Drawing for the job (mm, zero at the part's lowest x, y, z). A direction names the side the tool comes from. Give positions to 0.01 mm unless a question says otherwise; leave off trailing zeros. Use one line per item in the form item = value. Start each with the question number.
1) Tool access for the marked faces 4 and 5: list every direction of +Z, -Z, +X, -X, +Y, -Y with a clear straight run to the whole face (end or side of a thin tool).
2) Probe line 1 (Y direction, x = 7.5, z = 6.35) (1 decimal); line 2 (Y direction, x = 3.5, z = 6.25); line 3 (Z direction, x = 11.5, y = 7.75) (1 decimal). List the from-to ranges inside material, lowest first.
3) Mould opens along Y. For the marked faces 1, 2 and 3 say: pulls with the +Y half, pulls with the -Y half, needs draft (parallel to the pull), parting line crosses it, or undercut.
4) Drop flat-ended pins along their axis: P1, Ø5, axis at x = 2.5, y = 4.5, coming from the -Z side (1 decimal); P2, Ø6, axis at x = 17.5, z = 2.5, coming from the -Y side; P3, Ø3, axis at x = 9, z = 2, coming from the +Y side (1 decimal). Give the stop position or say it passes through.
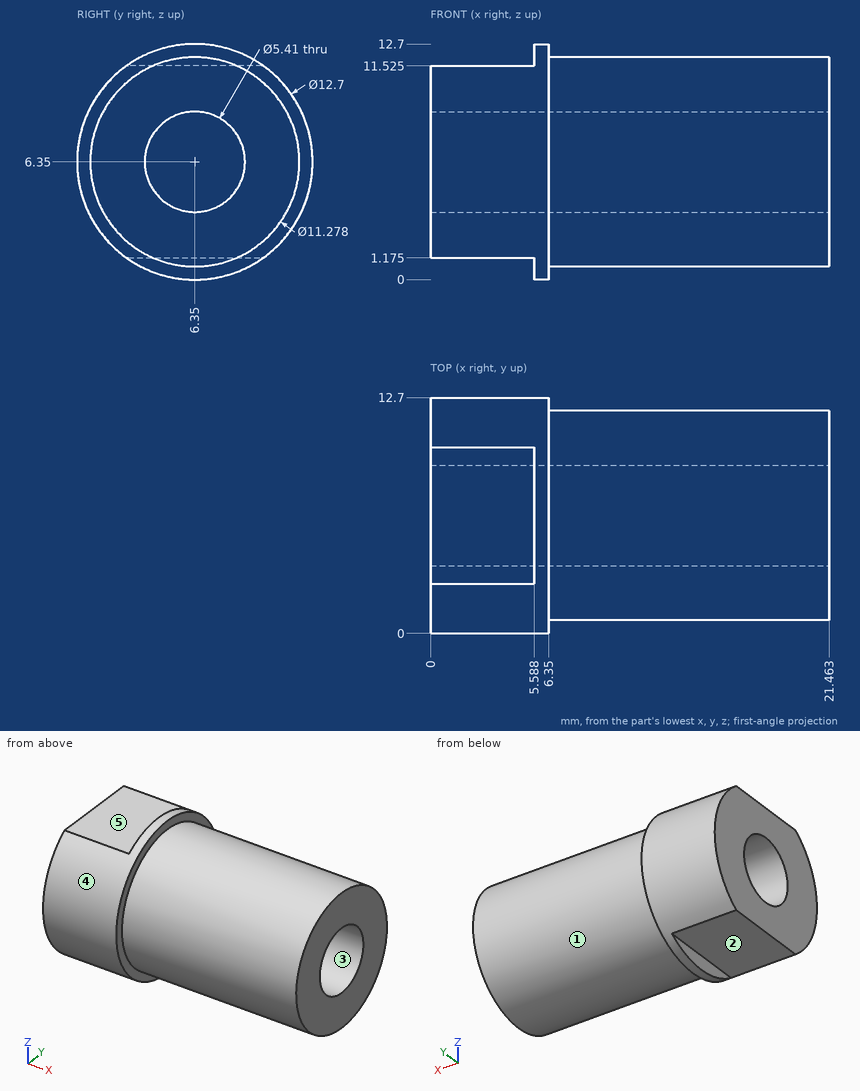
Result:
q1.face_4 = +X, -X
q1.face_5 = +Z, -X, +Y, -Y
q2.line_1 = 0.7 to 3.6, 9.1 to 12
q2.line_2 = 0 to 3.65, 9.05 to 12.7
q2.line_3 = 0.9 to 4, 8.7 to 11.8
q3.face_1 = parting line crosses it
q3.face_2 = needs draft
q3.face_3 = undercut
q4.P1 = 1.2
q4.P2 = 0.78
q4.P3 = 11.2
